Source: CAD feature listing. Evaluate the final solid. Frame: model axes, mm. Face numbers are marked on the shaded views. Round coordinates to 2 decimals unless told otherwise and drop trailing zeros. Order: outer loops, then holes, each group sorted by start corner. A loop starts at its lowest first (then second) coordinate and runs counter-clockwise, first axis right, second up. Notation, with made-up numbers: (-17, -31.5) -> (22, -31.5) arc R8 cw to (22, -22.5) -> close; hole circle Ø1 at (-38.5, 59.25). An arc over 180 degrees is marked (long way). Answer as CSV lines item,"result". Start each with the question number.
(1) Pull-direction query (X, two-part tool) for the marked faces 1 and 2; classes: +X half, -X half, draft (parallel to the pull), parting line (faces both ways), or undercut.
(2) Section query B-B (z = 131.5). Output: boundary loops of the cut face in (x, y) (3 decimals), plus the area to 3 significant figures.
(3) Section query C-C (y = 4.25). Output: boundary loops of the cut face in (x, z) (3 decimals), plus the area to 3 significant figures.
(4) Section query A-A (x = -9). Output: boundary loops of the cut face in (y, z) (3 decimals), plus the area to 3 significant figures.
(5) Line query: line 1 along Y through (x, z) = (-1, -20.5) (3 decimals); line 2 along X through (y, z) = (0.75, 131.5) (3 decimals). Output: solid intervals per line, ascending. Write a range as from..to.
(6) Contact query for a flat-ended pin moving along its axis: P1, Ø6, axis at x = -17.5, y = 7, coming from the +Z side. Output: stop coordinate, or through.
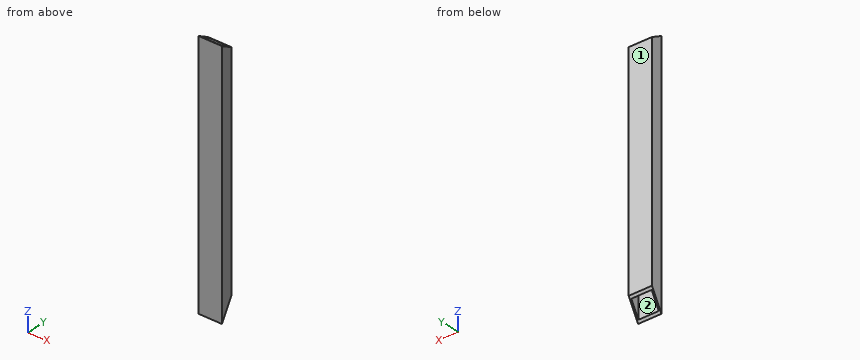
Autodesk Inventor part; units mm, degrees
ref_plane "YZ Plane" through (0, 0, 0) normal (1, 0, 0) x (0, 1, 0)
ref_plane "XZ Plane" through (0, 0, 0) normal (0, 1, 0) x (-1, 0, 0)
ref_plane "XY Plane" through (0, 0, 0) normal (0, 0, 1) x (1, 0, 0)
sketch "Sketch1" plane through (0, 0, 0) normal (0, 0, 1) x (1, 0, 0)
  line L0 (-35.56, 0) -> (35.56, 0)
  line L1 (0, -17.78) -> (0, 17.78)
  line L2 (-25.4, 12.7) -> (25.4, 12.7)
  line L3 (25.4, 12.7) -> (25.4, -12.7)
  line L4 (25.4, -12.7) -> (-25.4, -12.7)
  line L5 (-25.4, -12.7) -> (-25.4, 12.7)
  line L6 (22.225, 9.525) -> (-22.225, 9.525)
  line L7 (-22.225, 9.525) -> (-22.225, -9.525)
  line L8 (-22.225, -9.525) -> (22.225, -9.525)
  line L9 (22.225, -9.525) -> (22.225, 9.525)
  point P0 (0, 0)
  point P1 (-25.4, 0)
  point P2 (0, 12.7)
  dimension "d0" = 25.4
  dimension "d1" = 3.175
  dimension "d7" = 50.8
extrude "Base" add sketch "Sketch1" along normal mid plane 558.8 contours L5 L2 L1 L6 L7 L0 | L0 L7 L8 L1 L4 L5 | L1 L8 L9 L0 L3 L4 | L2 L3 L0 L9 L6 L1
sketch "Sketch3" plane through (25.4, -12.7, 279.4) normal (1, 0, 0) x (0, 0, -1)
  line L0 (0, 25.4) -> (0, 0)
  line L1 (0, 25.4) -> (558.8, 25.4)
  line L2 (0, 0) -> (14.6647, 25.4)
  point P0 (279.4, 12.7)
  dimension "d8" = 30
extrude "Extrusion3" cut sketch "Sketch3" against normal through all
sketch "Sketch4" plane through (25.4, -12.7, -279.4) normal (1, 0, 0) x (0, 0, -1)
  line L0 (0, 0) -> (0, 25.4)
  line L1 (-544.1353, 25.4) -> (0, 25.4)
  line L2 (0, 0) -> (-43.9941, 25.4)
  point P0 (-279.4, 12.7)
  dimension "d11" = 60
extrude "Extrusion4" cut sketch "Sketch4" against normal through all
properties part number "tubing_template_0.125" material "Aluminum-6061"
Answer block:
1,face 1,"draft"
1,face 2,"undercut"
2,outline,"(-25.4, -12.7) -> (25.4, -12.7) -> (25.4, 12.7) -> (-25.4, 12.7) -> close; hole (-22.225, -9.525) -> (22.225, -9.525) -> (22.225, 9.525) -> (-22.225, 9.525) -> close"
2,area,"444 mm2"
3,outline,"(-25.4, -250.042) -> (-22.225, -250.042) -> (-22.225, 269.614) -> (-25.4, 269.614) -> close; (22.225, -250.042) -> (25.4, -250.042) -> (25.4, 269.614) -> (22.225, 269.614) -> close"
3,area,"3,300 mm2"
4,outline,"(-12.7, -279.4) -> (-9.525, -273.901) -> (-9.525, 277.567) -> (-12.7, 279.4) -> close; (9.525, -240.905) -> (12.7, -235.406) -> (12.7, 264.735) -> (9.525, 266.568) -> close"
4,area,"3,360 mm2"
5,line 1,"-12.7..-9.525, 9.525..12.7"
5,line 2,"-25.4..-22.225, 22.225..25.4"
6,P1,"z = 266.57"
